The model under review builds one solid part; all positions refer to its coordinate system, in mm. A direction names the side the tool comes from. Round coordinates to 2 decimals unless told otherwise and drop trailing zeros. Loops run counter-clockwise (first coordinate to the right, second up) from the corner with the lowest first, then second, coordinate; pieces in that order, holes last. Notation, with made-up numbers: (2, 43.5) -> (37, 43.5) arc R36 ccw to (37, 80.5) -> close; hole circle Ø4 at (-34, 86). An arc over 180 degrees is marked (long way). Use CSV: the item, a comma, the result in double quotes. Start each with the question number.
```python
from build123d import *

# Parameters (mm, degrees)
SKETCH_1_W          = 100
SKETCH_1_H          = 80
EXTRUDE_1_DEPTH     = 3
SKETCH_2_R          = 1.6
CUT_EXTRUDE_1_DEPTH = 129.097619025
FILLET_1_R          = 30
FILLET_2_R          = 30
FILLET_3_R          = 3


with BuildPart() as part:
    # 草图1 → 凸台-拉伸1 (new body)
    with BuildSketch(Plane.XY):
        with Locations((50, -40)):
            Rectangle(SKETCH_1_W, SKETCH_1_H)
    extrude(amount=EXTRUDE_1_DEPTH)

    # 草图2 → 切除-拉伸1 (cut, through all)
    with BuildSketch(Plane.XY.offset(3)):
        with Locations((42.5, -10)):
            Circle(SKETCH_2_R)
        with Locations(Location((57.5, -10, 0), (0, 0, 180))):
            Circle(SKETCH_2_R)
        with Locations((57.5, -20)):
            Circle(SKETCH_2_R)
        with Locations(Location((42.5, -20, 0), (0, 0, 180))):
            Circle(SKETCH_2_R)
        with Locations((42.5, -60)):
            Circle(SKETCH_2_R)
        with Locations(Location((57.5, -60, 0), (0, 0, 180))):
            Circle(SKETCH_2_R)
        with Locations((57.5, -70)):
            Circle(SKETCH_2_R)
        with Locations(Location((42.5, -70, 0), (0, 0, 180))):
            Circle(SKETCH_2_R)
        with Locations((20, -32.5)):
            Circle(SKETCH_2_R)
        with Locations(Location((30, -32.5, 0), (0, 0, 180))):
            Circle(SKETCH_2_R)
        with Locations((30, -47.5)):
            Circle(SKETCH_2_R)
        with Locations(Location((20, -47.5, 0), (0, 0, 180))):
            Circle(SKETCH_2_R)
        with Locations((80, -47.5)):
            Circle(SKETCH_2_R)
        with Locations(Location((70, -47.5, 0), (0, 0, 180))):
            Circle(SKETCH_2_R)
        with Locations((70, -32.5)):
            Circle(SKETCH_2_R)
        with Locations(Location((80, -32.5, 0), (0, 0, 180))):
            Circle(SKETCH_2_R)
        with Locations((14, -65)):
            Circle(SKETCH_2_R)
        with Locations(Location((24, -65, 0), (0, 0, 180))):
            Circle(SKETCH_2_R)
        with Locations((24, -75)):
            Circle(SKETCH_2_R)
        with Locations(Location((14, -75, 0), (0, 0, 180))):
            Circle(SKETCH_2_R)
        with Locations((95, -4)):
            Circle(SKETCH_2_R)
        with Locations(Location((85, -4, 0), (0, 0, 180))):
            Circle(SKETCH_2_R)
        with Locations(Location((95, -14, 0), (0, 0, 180))):
            Circle(SKETCH_2_R)
        with Locations((85, -14)):
            Circle(SKETCH_2_R)
        Polygon((35, 0), (0, -30), (0, 0), align=None)
        Polygon((100, -80), (100, -50), (65, -80), align=None)
        Polygon((40, -34), (40, -46), (49, -46), align=None)
        Polygon((51, -34), (60, -46), (60, -34), align=None)
    extrude(amount=-CUT_EXTRUDE_1_DEPTH, mode=Mode.SUBTRACT)

    # 圆角1
    fillet_1_edges = [part.edges().sort_by_distance(p)[0] for p in [
        (0, -30, 1.5),
        (100, -50, 1.5),
    ]]
    fillet(fillet_1_edges, radius=FILLET_1_R)

    # 圆角2
    fillet_2_edges = [part.edges().sort_by_distance(p)[0] for p in [
        (35, 0, 1.5),
        (65, -80, 1.5),
    ]]
    fillet(fillet_2_edges, radius=FILLET_2_R)

    # 圆角3
    fillet_3_edges = [part.edges().sort_by_distance(p)[0] for p in [
        (100, 0, 1.5),
        (0, -80, 1.5),
    ]]
    fillet(fillet_3_edges, radius=FILLET_3_R)


solid = part.part
```
1. Take a section at C-C, the plane y = -47.5. Give the boundary of the cut face in (x, z).
2. The part is to be moulded in two halves that separate along X. For faces 1 (the face through (93.4, -3.93, 1.52)), 2 (the face through (35.55, -1.915, 1.479)), 3 (the face through (64.17, -78.19, 1.48)), say which applies: pulls with the +X half, pulls with the -X half, needs draft (parallel to the pull), parting line crosses it, or undercut.
3. Take a section at B-B, the plane y = -14. Give the boundary of the cut face in (x, z), then the cut area to 3 significant figures.
4. For faces 4 (the face through (44.56, -40.08, 1.52)), 5 (the face through (49, -39, 0)), list the 3-axis set-ups (+Z, -Z, +X, -X, +Y, -Y) from which the entire face can be reached by the end or side of a thin tool; tool diameter is ignored.
5. Take a section at A-A, the plane x = 95. Give the boundary of the cut face in (y, z).
6. Take a section at D-D, the plane z = 1.8. Count the separate pieces of the cut face and the enclosed holes in it, then the cut area to 3 significant figures.
7. Clearance check with flat-ended pins moving along their axes: P1, Ø5, axis at x = 95, y = -4, coming from the -Z side; P2, Ø0.9, axis at y = -39.5, z = 1.5, coming from the +X side. State where each tip first meets the part, or that it passes through.
8. For line 1 along Y through (x, z) = (58.5, 2.8); line 2 along X through (y, z) = (-64.5, 1.5); line 3 along Y through (x, z) = (14, 1.05), list the stretches that pass through material, from the lowest coordinate up. Write a range as from..to.
Results:
1,outline,"(0, 0) -> (18.4, 0) -> (18.4, 3) -> (0, 3) -> close; (21.6, 0) -> (28.4, 0) -> (28.4, 3) -> (21.6, 3) -> close; (31.6, 0) -> (68.4, 0) -> (68.4, 3) -> (31.6, 3) -> close; (71.6, 0) -> (78.4, 0) -> (78.4, 3) -> (71.6, 3) -> close; (81.6, 0) -> (97.79, 0) -> (97.79, 3) -> (81.6, 3) -> close"
2,face 1,"undercut"
2,face 2,"pulls with the -X half"
2,face 3,"pulls with the +X half"
3,outline,"(18.67, 0) -> (83.4, 0) -> (83.4, 3) -> (18.67, 3) -> close; (86.6, 0) -> (93.4, 0) -> (93.4, 3) -> (86.6, 3) -> close; (96.6, 0) -> (100, 0) -> (100, 3) -> (96.6, 3) -> close"
3,area,"225 mm²"
4,face 4,"+Z, -Z"
4,face 5,"-Z, +X, -X, +Y, -Y"
5,outline,"(-52.79, 0) -> (-15.6, 0) -> (-15.6, 3) -> (-52.79, 3) -> close; (-12.4, 0) -> (-5.6, 0) -> (-5.6, 3) -> (-12.4, 3) -> close; (-2.4, 0) -> (0, 0) -> (0, 3) -> (-2.4, 3) -> close"
6,separate pieces,"1"
6,enclosed holes,"26"
6,area,"6,570 mm²"
7,P1,"z = 0"
7,P2,"x = 99.86"
8,line 1,"-79.65..-71.25, -68.75..-61.25, -58.75..-44, -34..-21.25, -18.75..-11.25, -8.75..0"
8,line 2,"0..12.48, 15.52..22.48, 25.52..83.08"
8,line 3,"-80..-76.6, -73.4..-66.6, -63.4..-18"
